Source: CAD feature listing. Evaluate the final solid. Frame: model axes, mm. Face numbers are marked on the shaded views. A direction names the side the tool comes from. Give positions to 0.01 mm unless a question says otherwise; leave off trailing zeros. Order: outer loops, then holes, each group sorted by start corner. A loop starts at its lowest first (then second) coordinate and runs counter-clockwise, first axis right, second up.
```python
from build123d import *

# Parameters (mm, degrees)
F0_W      = 31.75
F0_H      = 31.75
F1_DEPTH  = 11.1252
F10_DEPTH = 6.35
F11_R     = 3.1749
F12_W     = 4.36372
F12_H     = 6.35
F12_H_2   = 31.75
F13_DEPTH = 17.4752
F14_W     = 4.7752
F14_H     = 4.36372
F15_DEPTH = 4.7752


# Not quite as in the source:
# - a fillet or chamfer is up to 0.001 mm smaller than in the source, because OpenCascade refuses the exact size


with BuildPart() as f1:
    # F0 (on Right) → F1 (new body)
    with BuildSketch(Plane.YZ):
        Rectangle(F0_W, F0_H)
    extrude(amount=F1_DEPTH)

    # F6: sweep along a path in F5
    with BuildLine(Plane.XZ.offset(12.7)) as f6_path:
        Line((11.1252, 9.525), (17.4752, 9.525))
        ThreePointArc((17.4752, 9.525), (21.0785384003, 10.4308096264), (23.8252, 12.9328865162))
        Line((23.8252, 12.9328865162), (25.1507334947, 14.9312034475))
    # F2 (on face) → F6 (sweep)
    with BuildSketch(Plane.YZ.offset(11.1252)):
        with BuildLine():
            ThreePointArc((-15.875, 12.7), (-12.7, 9.525), (-9.525, 12.7))
            ThreePointArc((-9.525, 12.7), (-10.4549359718, 14.9450640323), (-12.7000000057, 15.875))
            ThreePointArc((-12.7000000057, 15.875), (-14.9450640323, 14.9450640282), (-15.875, 12.7))
        make_face()
    sweep(path=f6_path.line)

    # F9: F1 across plane


with BuildPart() as f1_1:
    add(f1.part)
    add(f1.part.mirror(Plane(origin=(0, 0, 15.875), x_dir=(1, 0, 0), z_dir=(0, -1, 0))))

    # F2 (on face) → F10 (join)
    with BuildSketch(Plane.YZ.offset(11.1252)):
        with BuildLine():
            ThreePointArc((-9.525, -12.7), (-12.7, -9.525), (-15.875, -12.7))
            ThreePointArc((-15.875, -12.7), (-14.9450640303, -14.9450640303), (-12.7, -15.875))
            ThreePointArc((-12.7, -15.875), (-10.4549359697, -14.9450640303), (-9.525, -12.7))
        make_face()
        with BuildLine():
            ThreePointArc((12.7, -15.875), (14.9450640303, -14.9450640303), (15.875, -12.7))
            ThreePointArc((15.875, -12.7), (10.4549359697, -10.4549359697), (12.7, -15.875))
        make_face()
    extrude(amount=F10_DEPTH)

    # F11 (radius 3.175 in the source; OpenCascade refuses exactly that, so slightly less here)
    f11_edges = [f1_1.edges().sort_by_distance(p)[0] for p in [
        (5.5626, -15.875, 15.875),
        (5.5626, -15.875, -15.875),
        (5.5626, 15.875, -15.875),
        (5.5626, 15.875, 15.875),
    ]]
    fillet(f11_edges, radius=F11_R)

    # F12 (on face) → F13 (join)
    with BuildSketch(Plane(origin=(0, 0, 0), x_dir=(0, -1, 0), z_dir=(-1, 0, 0))):
        with Locations((0.6621663562, 19.05)):
            Rectangle(F12_W, F12_H)
        with Locations((0.6621663562, 0)):
            Rectangle(F12_W, F12_H_2)
    extrude(amount=F13_DEPTH)

    # F14 (on face) → F15 (join)
    with BuildSketch(Plane.XY.offset(22.225)):
        with Locations((-15.0876, -0.6621663562)):
            Rectangle(F14_W, F14_H)
    extrude(amount=F15_DEPTH)


solid = f1_1.part
```
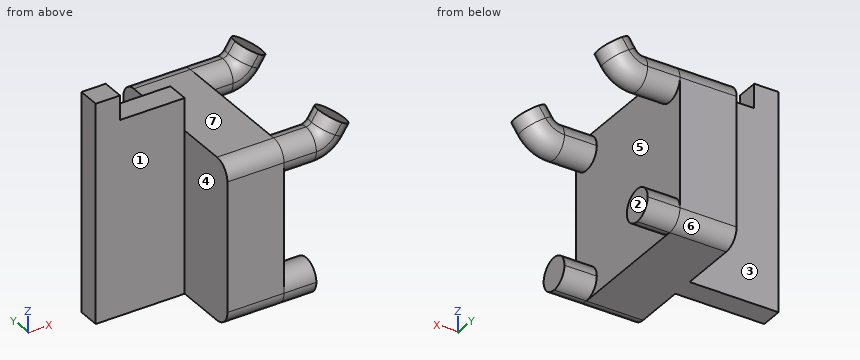
1) Material intervals for L1, parallel to X at y = -13, z = 5.5; L2, parallel to Z at x = 7.5, y = 11.5 (3 decimals); L3, parallel to Y at x = 13, z = 10, sorted ascending.
Report:
L1: x = 0 to 11.13
L2: z = -15.875 to 15.875
L3: y = -14.37 to -11.03, 11.03 to 14.37
2) Draft query along Z for the marked faces 4, 5, 6 and 7. Return one class per face: +Z half, -Z half, draft (parallel to the pull), parting line (faces both ways), or undercut.
Report:
face 4: draft
face 5: undercut
face 6: -Z half
face 7: +Z half
3) Section query D-D, the plane x = -6. Return the cut outline in (y, z) (3 decimals), and give its area (3 significant figures).
Report:
outline: (-2.844, -15.875) - (1.52, -15.875) - (1.52, 22.225) - (-2.844, 22.225) - close
area: 166 mm2
4) Section query A-A, the plane z = 8. Return the cut outline in (x, y) (3 decimals), and give its area (3 significant figures).
Report:
outline: (-17.475, -2.844) - (0, -2.844) - (0, -15.875) - (11.125, -15.875) - (11.125, 15.875) - (0, 15.875) - (0, 1.52) - (-17.475, 1.52) - close
area: 429 mm2
5) Pin query (flat end, axial travel): pin 1 (2 mm diameter, centred on y = 11.5, z = -10.5, fed in from -X); pin 2 (5 mm diameter, centred on x = 12.5, y = 4.5, fed in from +Z) (3 decimals); pin 3 (8.5 mm diameter, centred on x = -8.5, z = 15, fed in from -Y). Return the tip coordinate at first contact, or that it passes through.
Report:
pin 1: stops at x = 0
pin 2: stops at z = 15.875
pin 3: stops at y = -2.84
6) Section query C-C, the plane y = -3.5. Return the cut outline in (x, z) (3 decimals), and give its area (3 significant figures).
Report:
outline: (0, -15.875) - (11.125, -15.875) - (11.125, 15.875) - (0, 15.875) - close
area: 353 mm2
7) Reachability of the marked faces 1, 2 and 3 from +Z, -Z, +X, -X, +Y, -Y: full face, straight path, thin tool, end or side. Return the list, or none.
Report:
face 1: +Z, -Z, -X, -Y
face 2: -Z, +X, +Y, -Y
face 3: +Z, -Z, -X, +Y
8) Section query B-B, the plane x = 9. Return the cut outline in (y, z) (3 decimals).
Report:
outline: (-15.875, -12.7) arc R3.175 ccw to (-12.7, -15.875) - (12.7, -15.875) arc R3.175 ccw to (15.875, -12.7) - (15.875, 12.7) arc R3.175 ccw to (12.7, 15.875) - (-12.7, 15.875) arc R3.175 ccw to (-15.875, 12.7) - close
